Part model, mm, in its own coordinate system. A direction names the side the tool comes from. Coordinates: 2 decimals unless noted, no trailing zeros. Loops run counter-clockwise (first coordinate to the right, second up) from the corner with the lowest first, then second, coordinate; pieces in that order, holes last. Notation, with made-up numbers: M 29,60 L 47,60 A12 cw 47,83 Z; hole C -8.75,-15 d7. An arc over 180 degrees is marked long. Answer as CSV lines item,"result". Start each with the question number.
from build123d import *

# Parameters (mm, degrees)
EXTRUDE_2_DEPTH     = 4
EXTRUDE_3_DEPTH     = 51.85
EXTRUDE_4_DEPTH     = 51.85
SKETCH_6_W          = 32
SKETCH_6_H          = 27
SKETCH_6_W_2        = 3
CUT_EXTRUDE_1_DEPTH = 4
SKETCH_7_W          = 46
SKETCH_7_H          = 4
EXTRUDE_5_DEPTH     = 1.15
EXTRUDE_6_DEPTH     = 5
EXTRUDE_7_DEPTH     = 1
FILLET_3_R          = 2


with BuildPart() as part:
    # 草图1 → 凸台-拉伸2 (new body)
    with BuildSketch(Plane(origin=(0, 0, 0), x_dir=(1, 0, 0), z_dir=(0, 1, 0))):
        Polygon((16.85, -20.85), (17, -20.85), (17, 20.85), (16.85, 20.85), (-34.85, 20.85), (-34.85, -20.85), align=None)
        Polygon((17, -20.85), (17, -21), (31, -21), (35, -21), (35, -18), (35, 18), (35, 21), (31, 21), (17, 21), (17, 20.85), align=None)
        Polygon((31, -21), (17, -21), (17, -23), (37, -23), (37, 23), (17, 23), (17, 21), (31, 21), (35, 21), (35, 18), (35, -18), (35, -21), align=None)
    extrude(amount=EXTRUDE_2_DEPTH)

    # 草图4 → 凸台-拉伸3 (add)
    with BuildSketch(Plane.ZY.offset(-17)):
        Polygon((-20.85, 2), (-21.85, 1), (-20.85, 0), align=None)
    extrude(amount=EXTRUDE_3_DEPTH)

    # 草图3 → 凸台-拉伸4 (add)
    with BuildSketch(Plane.ZY.offset(-17)):
        Polygon((20.85, 2), (21.85, 1), (20.85, 0), align=None)
    extrude(amount=EXTRUDE_4_DEPTH)

    # 草图6 → 切除-拉伸1 (cut)
    with BuildSketch(Plane(origin=(0, 4, 0), x_dir=(1, 0, 0), z_dir=(0, 1, 0))):
        with Locations((-15.85, 0.35)):
            Rectangle(SKETCH_6_W, SKETCH_6_H)
        with Locations((-33.35, 0.35)):
            Rectangle(SKETCH_6_W_2, SKETCH_6_H)
    extrude(amount=-CUT_EXTRUDE_1_DEPTH, mode=Mode.SUBTRACT)

    # 草图7 → 凸台-拉伸5 (add)
    with BuildSketch(Plane(origin=(37, 0, 0), x_dir=(0, 0, -1), z_dir=(1, 0, 0))):
        with Locations((0, 2)):
            Rectangle(SKETCH_7_W, SKETCH_7_H)
    extrude(amount=EXTRUDE_5_DEPTH)

    # 草图12 → 凸台-拉伸6 (add, symmetric)
    with BuildSketch(Plane.XY):
        Polygon((36.65, 0), (36.65, -0.75), (37.4, 0), align=None)
        Polygon((35.9, 0), (36.65, -0.75), (36.65, 0), align=None)
    extrude(amount=EXTRUDE_6_DEPTH, both=True)

    # 草图14 → 凸台-拉伸7 (add)
    with BuildSketch(Plane.ZY.offset(34.85)):
        Polygon((-13.85, 0), (-13.85, 4), (-20.85, 4), (-20.85, 2), (-21.85, 1), (-20.85, 0), align=None)
    extrude(amount=EXTRUDE_7_DEPTH)

    # 圆角3
    fillet_3_edges = [part.edges().sort_by_distance(p)[0] for p in [
        (27.575, 4, 23),
        (27.575, 4, -23),
        (38.15, 2, 23),
        (38.15, 2, -23),
        (38.15, 4, 0),
    ]]
    fillet(fillet_3_edges, radius=FILLET_3_R)


solid = part.part
Q1. Wall check: L1, parallel to Z at x = -23, y = 3.6; L2, parallel to Z at x = -13.5, y = 1; L3, parallel to Z at x = 12, y = 3.8. Give the ranges that are in metal, low to high.
Q2. Slice it at C-C, the plane x = 2.5. Write the cut outline in (y, z), and give its area (3 significant figures).
Q3. Tool access for faces 5 (the face through (0.15, 2, 0)), 6 (the face through (-9, 3, 20.85)), 7 (the face through (-34.85, 2, 18)), 8 (the face through (-9, 3, -20.85)): list every direction of +Z, -Z, +X, -X, +Y, -Y with a clear straight run to the whole face (end or side of a thin tool).
Q4. Slice it at A-A, the plane x = -8.5. Write the cut outline in (y, z), and give its area (3 significant figures).
Q5. Flat gauge pins, fed straight in: P1, Ø0.6, axis at x = 37, y = -0.5, coming from the -Z side; P2, Ø2, axis at x = -24.5, y = 1.5, coming from the -Z side; P3, Ø1.1, axis at y = 3, z = -21.5, coming from the -X side. Where does each tip first touch, or does it go through?
Q6. Slice it at D-D, the plane y = 3.15. Write the cut outline in (x, z), and give its area (3 significant figures).
Q7. Slice it at B-B, the plane z = -0.5. Write the cut outline in (x, y).
Q8. Two-plate mould, pull along Z, no slides. Class faces 1 (the face through (17, 2, 22)), 2 (the face through (26, 1, 23)), 3 (the face through (-18, 2, -13.85)), 4 (the face through (-18, 2, 13.15)): +Z half, -Z half, draft (parallel to the pull), parting line (faces both ways), or undercut.
Solved:
1,L1,"z = -20.85 to -13.85, 13.15 to 20.85"
1,L2,"z = -21.85 to -13.85, 13.15 to 21.85"
1,L3,"z = -20.85 to 20.85"
2,outline,"M 0,-20.85 L 1,-21.85 L 2,-20.85 L 4,-20.85 L 4,20.85 L 2,20.85 L 1,21.85 L 0,20.85 Z"
2,area,"169 mm2"
3,face 5,"-X, +Y, -Y"
3,face 6,"+Z, -X, +Y"
3,face 7,"+Z, -X, +Y, -Y"
3,face 8,"-Z, -X, +Y"
4,outline,"M 0,-20.85 L 1,-21.85 L 2,-20.85 L 4,-20.85 L 4,-13.85 L 0,-13.85 Z; M 0,13.15 L 4,13.15 L 4,20.85 L 2,20.85 L 1,21.85 L 0,20.85 Z"
4,area,"60.8 mm2"
5,P1,"stops at z = -5"
5,P2,"stops at z = -21.85"
5,P3,"stops at x = 17"
6,outline,"M -35.85,-20.85 L 17,-20.85 L 17,-22.64 L 36.15,-22.64 A1.64 ccw 37.79,-21 L 37.79,21 A1.64 ccw 36.15,22.64 L 17,22.64 L 17,20.85 L -34.85,20.85 L -34.85,13.15 L 0.15,13.15 L 0.15,-13.85 L -35.85,-13.85 Z"
6,area,"2,160 mm2"
7,outline,"M 0.15,0 L 35.9,0 L 36.65,-0.75 L 37.4,0 L 38.15,0 L 38.15,2 A2 ccw 36.15,4 L 0.15,4 Z"
8,face 1,"draft"
8,face 2,"+Z half"
8,face 3,"undercut"
8,face 4,"undercut"
